Geometry check sheet. Reference: drawing and pictorial views, mm from the part's lowest x, y, z. A direction names the side the tool comes from. Round coordinates to 2 decimals unless told otherwise and drop trailing zeros. Write each loop counter-clockwise with the first axis right and the second up, starting at its lowest first coordinate (ties: lowest second). Pieces come first, ordered by that corner, then holes.
Item 1: Set-up check for the marked faces 1, 2, 3 and 4: record each of +Z, -Z, +X, -X, +Y, -Y from which the full face is reachable in a straight line by a thin tool's end or side.
Item 2: Section check A-A, the plane x = 42.15. Record the cut outline in (y, z).
Item 3: Section check C-C, the plane z = 44. Record the cut outline in (x, y) (3 decimals).
Item 4: Depth check by flat-ended pin: pin 1 (14 mm diameter, centred on y = 67, z = 38, fed in from +X) (3 decimals); pin 2 (2 mm diameter, centred on x = 32, y = 25.5, fed in from -Z); pin 3 (16 mm diameter, centred on y = 60.5, z = 40, fed in from -X) (3 decimals); pin 4 (5 mm diameter, centred on x = 27.5, z = 51.5, fed in from -Y). Enter the tip coordinate at first touch or a pass-through.
Item 5: Release check for a two-part mould opening along Y. For the marked faces 5, 6, 7 and 8 record: pulls with the +Y half, pulls with the -Y half, needs draft (parallel to the pull), parting line crosses it, or undercut.
Item 6: Material ranges on line 1 along Y through (x, z) = (12.6, 42.15); line 2 along Z through (x, y) = (68, 55); line 3 along X through (y, z) = (51, 55) (3 decimals), recorded low to high.
Item 7: Section check B-B, the plane y = 64. Record the cut outline in (x, z) (3 decimals), plus the area to 3 significant figures.
Item 8: Section check D-D, the plane x = 12. Record the cut outline in (y, z), plus the area to 3 significant figures.
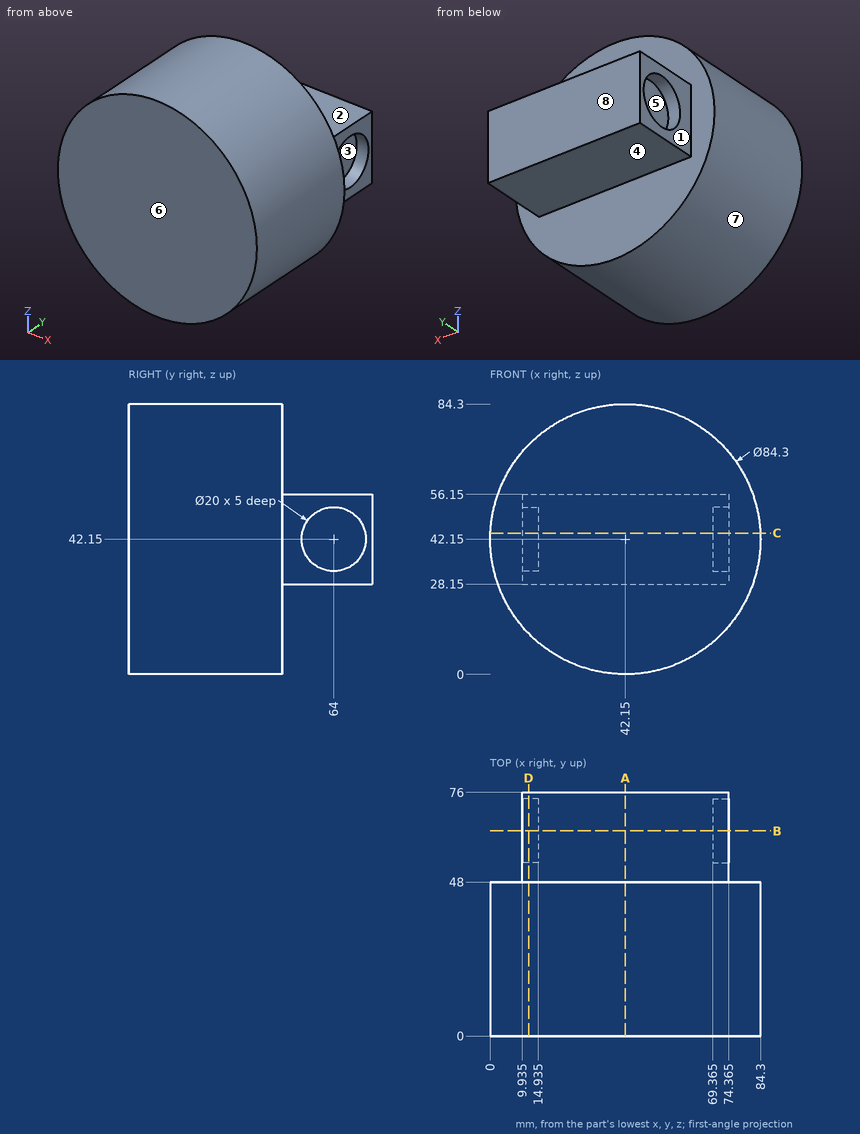
Values found:
1. face 1: +Z, -Z, -X, +Y
1. face 2: +Z, +X, -X, +Y
1. face 3: +X
1. face 4: -Z, +X, -X, +Y
2. outline: (0, 0) - (48, 0) - (48, 28.15) - (76, 28.15) - (76, 56.15) - (48, 56.15) - (48, 84.3) - (0, 84.3) - close
3. outline: (0.041, 0) - (84.259, 0) - (84.259, 48) - (74.365, 48) - (74.365, 54.173) - (69.365, 54.173) - (69.365, 73.827) - (74.365, 73.827) - (74.365, 76) - (9.935, 76) - (9.935, 73.827) - (14.935, 73.827) - (14.935, 54.173) - (9.935, 54.173) - (9.935, 48) - (0.041, 48) - close
4. pin 1: stops at x = 74.365
4. pin 2: stops at z = 1.01
4. pin 3: stops at x = 9.935
4. pin 4: stops at y = 0
5. face 5: undercut
5. face 6: pulls with the -Y half
5. face 7: needs draft
5. face 8: pulls with the +Y half
6. line 1: y = 0 to 54, 74 to 76
6. line 2: z = 28.15 to 56.15
6. line 3: x = 9.935 to 74.365
7. outline: (9.935, 28.15) - (74.365, 28.15) - (74.365, 32.15) - (69.365, 32.15) - (69.365, 52.15) - (74.365, 52.15) - (74.365, 56.15) - (9.935, 56.15) - (9.935, 52.15) - (14.935, 52.15) - (14.935, 32.15) - (9.935, 32.15) - close
7. area: 1,600 mm2
8. outline: (0, 12.69) - (48, 12.69) - (48, 28.15) - (76, 28.15) - (76, 56.15) - (48, 56.15) - (48, 71.61) - (0, 71.61) - close; hole circle Ø20 at (64, 42.15)
8. area: 3,300 mm2
